For this review, take the finished solid that the model builds, in its own axes (mm). Face numbers are marked on the shaded views. A direction names the side the tool comes from. Round coordinates to 2 decimals unless told otherwise and drop trailing zeros. Write each loop counter-clockwise with the first axis right and the second up, starting at its lowest first coordinate (ties: lowest second). Pieces come first, ordered by that corner, then holes. Notation, with made-up numbers: (-26.75, 72) - (13.25, 72) arc R22 cw to (13.25, 91) - close; hole circle Ø1 at (62.25, 59). An arc over 180 degrees is marked (long way). Answer in a Markdown table with one row per item. Add a question column.
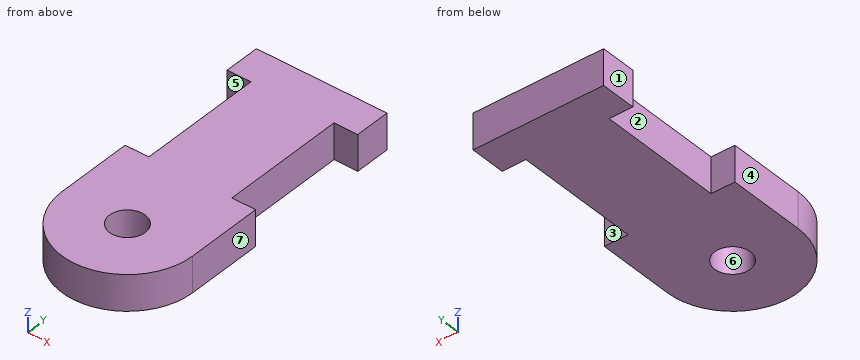
Autodesk Inventor part; units mm, degrees
ref_plane "YZ Plane" through (0, 0, 0) normal (1, 0, 0) x (0, 1, 0)
ref_plane "XZ Plane" through (0, 0, 0) normal (0, 1, 0) x (-1, 0, 0)
ref_plane "XY Plane" through (0, 0, 0) normal (0, 0, 1) x (1, 0, 0)
sketch "Sketch6" plane through (0, 0, 0) normal (0, 0, 1) x (1, 0, 0)
  line L0 (11, 25.4786) -> (0, 25.4786)
  line L1 (2, 22.4786) -> (2, 11.9786)
  line L2 (9, 22.4786) -> (9, 11.9786)
  line L3 (2, 11.9786) -> (0, 11.9786)
  line L4 (9, 11.9786) -> (11, 11.9786)
  arc A0 (0, 5.5) -> (11, 5.5) centre (5.5, 5.5) ccw
  circle A1 centre (5.5, 5.5) radius 1.5
  line L5 (0, 22.4786) -> (2, 22.4786)
  line L6 (9, 22.4786) -> (11, 22.4786)
  line L7 (0, 25.4786) -> (0, 22.4786)
  line L8 (0, 11.9786) -> (0, 5.5)
  line L9 (11, 5.5) -> (11, 11.9786)
  line L10 (11, 22.4786) -> (11, 25.4786)
  point P0 (0, 0)
  point P1 (10, 11.9786)
  dimension "d92" = 10.5
  dimension "d93" = 10.5
  dimension "d94" = 2
  dimension "d95" = 2
  dimension "d96" = 3
  dimension "d97" = 11
  dimension "d98" = 6.4786
extrude "Extrusion3" add sketch "Sketch6" along normal blind 3
properties part number "4P.01.02.27-BC-v1-Final Aileron L2 80deg" material "Acrylic, Clear"
Q1. Add section C-C on x = 5.5. State the section outline as (y, z) points, then the cut area to 3 significant figures.
Q2. Add section D-D on y = 15. State the section outline as (x, z) points.
Q3. To check wall thickness, follow probe 1 along Y at (x, z) = (5.5, 1); probe 2 along X at (y, z) = (4.25, 2); probe 3 along X at (y, z) = (15.5, 1.5). State the ranges of each line that lie inside material, in increasing order.
Q4. Draft analysis for pull direction X (two halves, no side actions). For the marked faces 4, 5, 6 and 7, state which applies: released by +X, released by -X, zero draft, split by the parting line, or undercut.
Q5. Tool access review of the marked faces 1, 2 and 3: name each direction out of +Z, -Z, +X, -X, +Y, -Y from which nothing blocks a thin tool from reaching the whole face with its end or side.
Q6. Add section B-B on z = 1.75. State the section outline as (x, y) points.
Q7. Add section A-A on x = 6.75. State the section outline as (y, z) points, then the cut area to 3 significant figures.
Q8. Insertion check: pin 1 Ø1.5 at (x, y) = (3, 18.5) entering from -Z; pin 2 Ø1.5 at (y, z) = (14.5, 1) entering from -X; pin 3 Ø0.6 at (x, z) = (0.5, 2) entering from -Y. Each pin has a flat end and moves straight along its axis. Give the tip position at first contact, or say it passes through.
Answer sheet:
| question | item | result |
|---|---|---|
| 1 | outline | (0, 0) - (4, 0) - (4, 3) - (0, 3) - close; (7, 0) - (25.48, 0) - (25.48, 3) - (7, 3) - close |
| 1 | area | 67.4 mm² |
| 2 | outline | (2, 0) - (9, 0) - (9, 3) - (2, 3) - close |
| 3 | probe 1 | y = 0 to 4, 7 to 25.48 |
| 3 | probe 2 | x = 0.14 to 4.67, 6.33 to 10.86 |
| 3 | probe 3 | x = 2 to 9 |
| 4 | face 4 | released by -X |
| 4 | face 5 | zero draft |
| 4 | face 6 | undercut |
| 4 | face 7 | released by +X |
| 5 | face 1 | +Z, -Z, -X, +Y, -Y |
| 5 | face 2 | +Z, -Z, -X |
| 5 | face 3 | +Z, -Z, +X |
| 6 | outline | (0, 5.5) arc R5.5 ccw to (11, 5.5) - (11, 11.98) - (9, 11.98) - (9, 22.48) - (11, 22.48) - (11, 25.48) - (0, 25.48) - (0, 22.48) - (2, 22.48) - (2, 11.98) - (0, 11.98) - close; hole circle Ø3 at (5.5, 5.5) |
| 7 | outline | (0.14, 0) - (4.67, 0) - (4.67, 3) - (0.14, 3) - close; (6.33, 0) - (25.48, 0) - (25.48, 3) - (6.33, 3) - close |
| 7 | area | 71.0 mm² |
| 8 | pin 1 | stops at z = 0 |
| 8 | pin 2 | stops at x = 2 |
| 8 | pin 3 | stops at y = 2.64 |
